Model file for the job. Use its own axes, mm. A direction names the side the tool comes from. Give positions to 0.01 mm unless a question says otherwise; leave off trailing zeros. Write each loop counter-clockwise with the first axis right and the second up, starting at its lowest first coordinate (ties: lowest second). Pieces come first, ordered by that corner, then holes. Notation, with made-up numbers: (81, -13.5) - (138, -13.5) arc R23 cw to (138, 4.5) - close; hole circle Ø7 at (6.25, -36.5). An arc over 180 degrees is marked (long way). Use CSV: the item, a comma, the result in double quotes.
from build123d import *

# Parameters (mm, degrees)
SKETCH1_R           = 3.1
SKETCH1_R_2         = 2.5
BOSS_EXTRUDE1_DEPTH = 15
SKETCH6_R           = 3.1
BOSS_EXTRUDE3_DEPTH = 5
BOSS_EXTRUDE4_DEPTH = 15
SKETCH8_R           = 2.5
CUT_EXTRUDE3_DEPTH  = 25
CUT_EXTRUDE4_DEPTH  = 16
SKETCH11_W          = 24
SKETCH11_H          = 0.25
BOSS_EXTRUDE5_DEPTH = 15
SKETCH12_W          = 24
SKETCH12_H          = 32
SKETCH12_H_2        = 23
BOSS_EXTRUDE6_DEPTH = 22
SKETCH13_R          = 6.1
CUT_EXTRUDE5_DEPTH  = 25


with BuildPart() as part:
    # Sketch1 → Boss-Extrude1 (new body)
    with BuildSketch(Plane.XY):
        with BuildLine():
            Line((-25.80048806, 37.524276553), (-49.80048806, 37.524276553))
            Line((-49.80048806, 37.524276553), (-49.80048806, -14.975723447))
            Line((-49.80048806, -14.975723447), (-41.80048806, -45.286414829))
            ThreePointArc((-41.80048806, -45.286414829), (-37.80048806, -49.286414829), (-33.80048806, -45.286414829))
            Line((-33.80048806, -45.286414829), (-25.80048806, -14.975723447))
            Line((-25.80048806, -14.975723447), (-25.80048806, 37.524276553))
        make_face()
        with Locations((-37.80048806, 25.524276553)):
            Circle(SKETCH1_R, mode=Mode.SUBTRACT)
        with Locations((-37.80048806, -2.975723447)):
            Circle(SKETCH1_R, mode=Mode.SUBTRACT)
        with Locations((-37.80048806, -45.286414829)):
            Circle(SKETCH1_R_2, mode=Mode.SUBTRACT)
    extrude(amount=BOSS_EXTRUDE1_DEPTH)

    # Sketch6 → Boss-Extrude3 (add)
    with BuildSketch(Plane.XY.offset(15)):
        with Locations((-37.80048806, -2.975723447)):
            Circle(SKETCH6_R)
        with Locations((-37.80048806, 25.524276553)):
            Circle(SKETCH6_R)
    extrude(amount=-BOSS_EXTRUDE3_DEPTH)

    # Sketch7 → Boss-Extrude4 (add)
    with BuildSketch(Plane.XY.offset(15)):
        Polygon((-51.800511672, 16.774276553), (-49.80048806, 16.774276553), (-49.80048806, -15.225723447), (-72.300511672, -15.225723447), (-72.300511672, 16.774276553), (-64.300511672, 16.774276553), (-64.300511672, -7.225723447), (-58.050499866, -7.225723447), (-51.800511672, -7.225723447), align=None)
    extrude(amount=-BOSS_EXTRUDE4_DEPTH)

    # Sketch8 → Cut-Extrude3 (cut)
    with BuildSketch(Plane.ZY.offset(72.300511672)):
        with Locations((7.5, 8.346782821)):
            Circle(SKETCH8_R)
    extrude(amount=-CUT_EXTRUDE3_DEPTH, mode=Mode.SUBTRACT)

    # Sketch10 → Cut-Extrude4 (cut, through all)
    with BuildSketch(Plane.XY.offset(15)):
        Polygon((-49.80048806, -15.225723447), (-49.80048806, -14.975723447), (-25.80048806, -14.975723447), (-25.80048806, -50.615055613), (-49.80048806, -50.615055613), align=None)
    extrude(amount=-CUT_EXTRUDE4_DEPTH, mode=Mode.SUBTRACT)

    # Sketch11 → Boss-Extrude5 (add)
    with BuildSketch(Plane.XY.offset(15)):
        with Locations((-37.80048806, -15.100723447)):
            Rectangle(SKETCH11_W, SKETCH11_H)
    extrude(amount=-BOSS_EXTRUDE5_DEPTH)

    # Sketch12 → Boss-Extrude6 (add)
    with BuildSketch(Plane.XY.offset(15)):
        with Locations((-37.80048806, 0.774276553)):
            Rectangle(SKETCH12_W, SKETCH12_H)
        with Locations((-37.80048806, -26.725723447)):
            Rectangle(SKETCH12_W, SKETCH12_H_2)
    extrude(amount=BOSS_EXTRUDE6_DEPTH)

    # Sketch13 → Cut-Extrude5 (cut, through all)
    with BuildSketch(Plane.ZY.offset(49.80048806)):
        with Locations((26, 3.274276553)):
            Circle(SKETCH13_R)
        with Locations((26, -24.725723447)):
            Circle(SKETCH13_R)
    extrude(amount=-CUT_EXTRUDE5_DEPTH, mode=Mode.SUBTRACT)


solid = part.part
(1) Pull direction Y, two halves, no side cores. Call faces 5 (the face through (-25.8, -1, 18)), 6 (the face through (-58, -7.226, 8)), 7 (the face through (-37.968, -24.458, 19.906)): released by +Y, released by -Y, zero draft, split by the parting line, or undercut.
Checked values:
face 5,"zero draft"
face 6,"released by +Y"
face 7,"undercut"
(2) Wall check: probe 1 along Y at (x, z) = (-44, 26); probe 2 along X at (y, z) = (11, 8); probe 3 along X at (y, z) = (-4, 6). Give the ranges that are in metal, low to high. Write a range as [from, to].
Checked values:
probe 1,"y = [-38.23, -30.83], [-18.63, -2.83], [9.37, 16.77]"
probe 2,"x = [-72.3, -64.3], [-51.8, -25.8]"
probe 3,"x = [-72.3, -64.3], [-51.8, -40.73], [-34.87, -25.8]"
(3) Saw through at C-C, the plane y = -27. List the corners of the cut face in (x, z).
Checked values:
outline,"(-49.8, 15) - (-25.8, 15) - (-25.8, 20.34) - (-49.8, 20.34) - close; (-49.8, 31.66) - (-25.8, 31.66) - (-25.8, 37) - (-49.8, 37) - close"
(4) Saw through at A-A, the plane z = 26. List the corners of the cut face in (x, y), then the cut area to 3 significant figures.
Checked values:
outline,"(-49.8, -38.23) - (-25.8, -38.23) - (-25.8, -30.83) - (-49.8, -30.83) - close; (-49.8, -18.63) - (-25.8, -18.63) - (-25.8, -2.83) - (-49.8, -2.83) - close; (-49.8, 9.37) - (-25.8, 9.37) - (-25.8, 16.77) - (-49.8, 16.77) - close"
area,"734 mm^2"
(5) Saw through at D-D, the plane x = -62. List the corners of the cut face in (y, z), then the cut area to 3 significant figures.
Checked values:
outline,"(-15.23, 0) - (-7.23, 0) - (-7.23, 15) - (-15.23, 15) - close"
area,"120 mm^2"
(6) Saw through at B-B, the plane z = 7.5. List the corners of the cut face in (x, y).
Checked values:
outline,"(-72.3, -15.23) - (-25.8, -15.23) - (-25.8, 37.52) - (-49.8, 37.52) - (-49.8, 16.77) - (-51.8, 16.77) - (-51.8, 10.85) - (-47.3, 10.85) - (-47.3, 5.85) - (-51.8, 5.85) - (-51.8, -7.23) - (-64.3, -7.23) - (-64.3, 5.85) - (-72.3, 5.85) - close; (-72.3, 10.85) - (-64.3, 10.85) - (-64.3, 16.77) - (-72.3, 16.77) - close; hole circle Ø6.2 at (-37.8, -2.98); hole circle Ø6.2 at (-37.8, 25.52)"
(7) 3-axis set-ups, long thin cutter, end or side, ignore diameter. For faces 1 (the face through (-38, 26, 10)), 2 (the face through (-68.36, 7.39, 9.81)), 3 (the face through (-49.8, 27, 7)), 4 (the face through (-66, -3, 15)): which of +Z, -Z, +X, -X, +Y, -Y reach the whole face in a straight line?
Checked values:
face 1,"-Z"
face 2,"-X"
face 3,"+Z, -Z, -X, +Y"
face 4,"+Z, -X, +Y, -Y"
(8) Flat gauge pins, fed straight in: P1, Ø6, axis at x = -45.5, y = -9, coming from the -Z side; P2, Ø5, axis at x = -37.8, y = 25.52, coming from the -Z side; P3, Ø14, axis at x = -60.5, z = 10, coming from the +Y side; P4, Ø6, axis at x = -37, y = 31, coming from the +Z side. Where does each tip first touch, or does it go through?
Checked values:
P1,"stops at z = 0"
P2,"stops at z = 10"
P3,"stops at y = 16.77"
P4,"stops at z = 15"
